from build123d import *

# Parameters (mm, degrees)
BOSS_EXTRUDE1_DEPTH = 50


with BuildPart() as part:
    # Sketch1 → Boss-Extrude1 (new body)
    with BuildSketch(Plane(origin=(0, 0, 0), x_dir=(1, 0, 0), z_dir=(0, 1, 0))):
        Polygon((-490.415824699, -64.194072769), (-472.477870031, -524.138824529), (-270.660991621, -696.876695154), (273.24324441, -696.876695154), (475.06012282, -524.138824529), (492.998077488, -64.194072769), (436.803486749, 330.511591748), (255.52688097, 580.827312496), (1.291126394, 709.058947943), (-252.944628181, 580.827312496), (-434.22123396, 330.511591748), align=None)
        with BuildLine():
            Line((198.047881985, -498.167821548), (-198.047881985, -498.167821548))
            Line((-198.047881985, -498.167821548), (-277.326571574, -430.312089493))
            Line((-277.326571574, -430.312089493), (-292.42397797, -43.20146483))
            ThreePointArc((-292.42397797, -43.20146483), (-211.574023689, 174.749059805), (0, 271.058866137))
            ThreePointArc((0, 271.058866137), (211.574023689, 174.749059805), (292.42397797, -43.20146483))
            Line((292.42397797, -43.20146483), (277.326571574, -430.312089493))
            Line((277.326571574, -430.312089493), (198.047881985, -498.167821548))
        make_face(mode=Mode.SUBTRACT)
    extrude(amount=-BOSS_EXTRUDE1_DEPTH)


solid = part.part
Input: part model. Units: mm. Frame: model coordinates. A direction names the side the tool comes from. Coordinates: 2 decimals unless noted, no trailing zeros. Loops run counter-clockwise (first coordinate to the right, second up) from the corner with the lowest first, then second, coordinate; pieces in that order, holes last. Notation, with made-up numbers: (-22, 49) -> (34, 49) arc R18 cw to (34, 59) -> close; hole circle Ø9 at (79.25, 81). An arc over 180 degrees is marked (long way). One line per item, written item: value.
(1) Ray query, line 1 along X through (y, z) = (-14.5, 305.5); line 2 along X through (y, z) = (-39, 295); line 3 along Z through (x, y) = (195, -39). Return the intervals inside material, ascending.
Answer below:
line 1: x = -481 to -282.19, 282.19 to 483.59
line 2: x = -481.41 to -282.6, 282.6 to 484
line 3: z = -611.36 to -191.24, 498.17 to 696.88
(2) Cut plane B-B (x = 69.5). Output: boundary loops of the cut face in (y, z).
Answer below:
outline: (-50, -674.66) -> (0, -674.66) -> (0, -260.6) -> (-50, -260.6) -> close; (-50, 498.17) -> (0, 498.17) -> (0, 696.88) -> (-50, 696.88) -> close
(3) Draft query along X for faces 3 (the face through (-284.77, -24.65, 239.47)), 4 (the face through (-124.05, -24.65, -645.84)), 5 (the face through (483.904, -24.65, 297.386)). Return one class per face: pulls with the +X half, pulls with the -X half, needs draft (parallel to the pull), parting line crosses it, or undercut.
Answer below:
face 3: undercut
face 4: pulls with the -X half
face 5: pulls with the +X half
(4) Cut plane C-C (z = -37). Output: boundary loops of the cut face in (x, y), then the cut area to 3 significant figures.
Answer below:
outline: (-476.01, -50) -> (-284.82, -50) -> (-284.82, 0) -> (-476.01, 0) -> close; (284.82, -50) -> (478.59, -50) -> (478.59, 0) -> (284.82, 0) -> close
area: 19,200 mm2
(5) Set-up query: faces 1 (the face through (-224, -50, -172)), 2 (the face through (3, -25, 498.168)). Return all of +Z, -Z, +X, -X, +Y, -Y with unobstructed straight access to the full face (end or side cutting, diameter ignored); none if empty.
Answer below:
face 1: +Z, -Z, +X, -X, -Y
face 2: +Y, -Y
(6) Pin query (flat end, axial travel): pin 1 Ø3 at (x, y) = (159.5, -30.5) entering from -Z; pin 2 Ø12 at (y, z) = (-33, -534) entering from -X; pin 3 Ø25 at (x, y) = (-20.5, -34) entering from -Z. Return the tip coordinate at first contact, or that it passes through.
Answer below:
pin 1: stops at z = -630.02
pin 2: stops at x = -291.2
pin 3: stops at z = -704.37
(7) Cut plane A-A (y = -20). Output: boundary loops of the cut face in (x, z).
Answer below:
outline: (-490.42, 64.19) -> (-434.22, -330.51) -> (-252.94, -580.83) -> (1.29, -709.06) -> (255.53, -580.83) -> (436.8, -330.51) -> (493, 64.19) -> (475.06, 524.14) -> (273.24, 696.88) -> (-270.66, 696.88) -> (-472.48, 524.14) -> close; hole (-292.42, 43.2) arc R302.63 ccw to (0, -271.06) arc R302.63 ccw to (292.42, 43.2) -> (277.33, 430.31) -> (198.05, 498.17) -> (-198.05, 498.17) -> (-277.33, 430.31) -> close
(8) Cut plane D-D (z = -448). Output: boundary loops of the cut face in (x, y), then the cut area to 3 significant figures.
Answer below:
outline: (-349.14, -50) -> (351.72, -50) -> (351.72, 0) -> (-349.14, 0) -> close
area: 35,000 mm2
